Input: part model. Units: mm. Frame: model coordinates. A direction names the side the tool comes from. Give positions to 0.01 mm unless a question says otherwise; leave off trailing zeros. Loops run counter-clockwise (first coordinate to the right, second up) from the corner with the lowest first, then second, coordinate; pieces in that order, holes last. Notation, with made-up numbers: (58, 76) -> (93, 76) arc R23 cw to (93, 86) -> close; hole circle Ø9 at (67, 4). An arc over 180 degrees is marked (long way). Answer in a Markdown table with one row per item. Add a question column.
```python
from build123d import *

# Parameters (mm, degrees)
SKETCH1_R           = 14.2875
SKETCH1_R_2         = 6.35
BOSS_EXTRUDE1_DEPTH = 7.9248
CHAMFER1_SIZE       = 1.27
SKETCH2_R           = 15.5575
SKETCH2_R_2         = 6.35
BOSS_EXTRUDE2_DEPTH = 1.524


with BuildPart() as part:
    # Sketch1 → Boss-Extrude1 (new body)
    with BuildSketch(Plane(origin=(0, 0, 0), x_dir=(1, 0, 0), z_dir=(0, 1, 0))):
        with Locations(Location((0, 0, 0), (0, 0, 270))):
            Circle(SKETCH1_R)
        with Locations(Location((0, 0, 0), (0, 0, 270))):
            Circle(SKETCH1_R_2, mode=Mode.SUBTRACT)
    extrude(amount=BOSS_EXTRUDE1_DEPTH)

    # Chamfer1
    chamfer1_edges = [part.edges().sort_by_distance(p)[0] for p in [
        (0, 7.9248, -14.2875),
    ]]
    chamfer(chamfer1_edges, length=CHAMFER1_SIZE)

    # Sketch2 → Boss-Extrude2 (add)
    with BuildSketch(Plane.XZ):
        with Locations(Location((0, 0, 0), (0, 0, 270))):
            Circle(SKETCH2_R)
        with Locations(Location((0, 0, 0), (0, 0, 90))):
            Circle(SKETCH2_R_2, mode=Mode.SUBTRACT)
    extrude(amount=-BOSS_EXTRUDE2_DEPTH)


solid = part.part
```
1) Section B-B on z = 0. Output: boundary loops of the cut face in (x, y), and give its area (3 significant figures).
2) Section A-A on x = 0. Output: boundary loops of the cut face in (y, z), and give its area (3 significant figures).
3) Reachability of faces 4 (the face through (-7, 0, 0)), 5 (the face through (0.628, 4.053, -14.274)) from +Z, -Z, +X, -X, +Y, -Y: full face, straight path, thin tool, end or side. Return the list, or none.
4) Section D-D on y = 7.25. Output: boundary loops of the cut face in (x, z), and give its area (3 significant figures).
5) Pin query (flat end, axial travel): pin 1 (3 mm diameter, centred on x = 12, z = 10, fed in from +Y); pin 2 (1 mm diameter, centred on x = -7.5, y = 4.5, fed in from -Z); pin 3 (1 mm diameter, centred on y = 1, z = -7, fed in from +X). Return the tip coordinate at first contact, or that it passes through.
6) Material intervals for line 1 along X through (y, z) = (4, 0); line 2 along X through (y, z) = (7.5, 5); line 3 along X through (y, z) = (6.5, 13), sorted ascending.
7) Pull-direction query (Z, two-part tool) for faces 1 (the face through (-3.86, 3.91, -5.04)), 2 (the face through (-13, 1.524, -7)), 3 (the face through (4.67, 0.75, -14.84)); classes: +Z half, -Z half, draft (parallel to the pull), parting line (faces both ways), or undercut.
Working result:
| question | item | result |
|---|---|---|
| 1 | outline | (-15.56, 0) -> (-6.35, 0) -> (-6.35, 7.92) -> (-13.02, 7.92) -> (-14.29, 6.65) -> (-14.29, 1.52) -> (-15.56, 1.52) -> close; (6.35, 0) -> (15.56, 0) -> (15.56, 1.52) -> (14.29, 1.52) -> (14.29, 6.65) -> (13.02, 7.92) -> (6.35, 7.92) -> close |
| 1 | area | 128 mm2 |
| 2 | outline | (0, -15.56) -> (1.52, -15.56) -> (1.52, -14.29) -> (6.65, -14.29) -> (7.92, -13.02) -> (7.92, -6.35) -> (0, -6.35) -> close; (0, 6.35) -> (7.92, 6.35) -> (7.92, 13.02) -> (6.65, 14.29) -> (1.52, 14.29) -> (1.52, 15.56) -> (0, 15.56) -> close |
| 2 | area | 128 mm2 |
| 3 | face 4 | +Z, -Z, +X, -X, -Y |
| 3 | face 5 | +Y |
| 4 | outline | circle Ø27.38 at (0, 0); hole circle Ø12.7 at (0, 0) |
| 4 | area | 462 mm2 |
| 5 | pin 1 | stops at y = 6.82 |
| 5 | pin 2 | stops at z = -12.46 |
| 5 | pin 3 | stops at x = 14.13 |
| 6 | line 1 | x = -14.29 to -6.35, 6.35 to 14.29 |
| 6 | line 2 | x = -12.48 to -3.91, 3.91 to 12.48 |
| 6 | line 3 | x = -5.93 to 5.93 |
| 7 | face 1 | undercut |
| 7 | face 2 | draft |
| 7 | face 3 | parting line |
